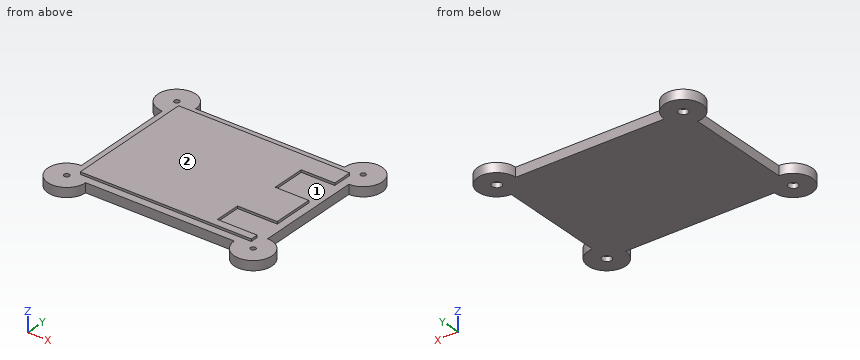
```python
from build123d import *

# Parameters (mm, degrees)
SKETCH024_W     = 79
SKETCH024_H     = 61
PAD006_DEPTH    = 4
SKETCH025_W     = 72.5
SKETCH025_H     = 54.5
PAD007_DEPTH    = 1
SKETCH026_W     = 14.223953
SKETCH026_H     = 14.414499
SKETCH026_W_2   = 16.850891
SKETCH026_H_2   = 11.145231
POCKET015_DEPTH = 1
SKETCH029_R     = 8
PAD010_DEPTH    = 4
SKETCH030_R     = 1.1
POCKET016_DEPTH = 5.001
SKETCH031_R     = 2
POCKET017_DEPTH = 2


with BuildPart() as part:
    # Sketch024 → Pad006 (new body)
    with BuildSketch(Plane.XY):
        Rectangle(SKETCH024_W, SKETCH024_H)
    extrude(amount=-PAD006_DEPTH)

    # Sketch025 (on Face5 of Pad006) → Pad007 (join)
    with BuildSketch(Plane.XY):
        Rectangle(SKETCH025_W, SKETCH025_H)
    extrude(amount=PAD007_DEPTH)

    # Sketch026 (on Face11 of Pad007) → Pocket015 (cut)
    with BuildSketch(Plane.XY.offset(1)):
        with Locations((29.1380235, 11.7657555)):
            Rectangle(SKETCH026_W, SKETCH026_H)
        with Locations((27.8245545, -18.4755795)):
            Rectangle(SKETCH026_W_2, SKETCH026_H_2)
    extrude(amount=-POCKET015_DEPTH, mode=Mode.SUBTRACT)

    # Sketch029 (on Face5 of Pocket015) → Pad010 (join)
    with BuildSketch(Plane(origin=(0, 0, -4), x_dir=(1, 0, 0), z_dir=(0, 0, -1))):
        with Locations((39.5, 30.5)):
            Circle(SKETCH029_R)
        with Locations((39.5, -30.5)):
            Circle(SKETCH029_R)
        with Locations((-39.5, -30.5)):
            Circle(SKETCH029_R)
        with Locations((-39.5, 30.5)):
            Circle(SKETCH029_R)
    extrude(amount=-PAD010_DEPTH)

    # Sketch030 (on Face20 of Pad010) → Pocket016 (cut, through all)
    with BuildSketch(Plane(origin=(0, 0, -4), x_dir=(1, 0, 0), z_dir=(0, 0, -1))):
        with Locations((39.5, 30.5)):
            Circle(SKETCH030_R)
        with Locations((39.5, -30.5)):
            Circle(SKETCH030_R)
        with Locations((-39.5, -30.5)):
            Circle(SKETCH030_R)
        with Locations((-39.5, 30.5)):
            Circle(SKETCH030_R)
    extrude(amount=-POCKET016_DEPTH, mode=Mode.SUBTRACT)

    # Sketch031 (on Face22 of Pocket016) → Pocket017 (cut)
    with BuildSketch(Plane(origin=(0, 0, -4), x_dir=(1, 0, 0), z_dir=(0, 0, -1))):
        with Locations((-39.5, 30.5)):
            Circle(SKETCH031_R)
        with Locations((-39.5, -30.5)):
            Circle(SKETCH031_R)
        with Locations((39.5, 30.5)):
            Circle(SKETCH031_R)
        with Locations((39.5, -30.5)):
            Circle(SKETCH031_R)
    extrude(amount=-POCKET017_DEPTH, mode=Mode.SUBTRACT)


with BuildPart() as part_1:
    # Body002 placement: moved
    add(part.part.moved(Location((0, 0, -17))))


solid = part_1.part
```
Design review of the part built by this model. Coordinates are the model's own, in mm. Face numbers are marked on the shaded views. Coordinates: 2 decimals unless noted, no trailing zeros. Order: outer loops, then holes, each group sorted by start corner. A loop starts at its lowest first (then second) coordinate and runs counter-clockwise, first axis right, second up.
1) Clearance check with flat-ended pins moving along their axes: pin 1 (1.1 mm diameter, centred on y = -0.5, z = -16.5, fed in from +X); pin 2 (0.5 mm diameter, centred on y = -9, z = -16.5, fed in from -X); pin 3 (3 mm diameter, centred on y = 3, z = -19.5, fed in from -X). State where each tip first meets the part, or that it passes through.
2) Wall thickness on line 1 along X through (y, z) = (6.5, -20); line 2 along Y through (x, z) = (14.5, -17.15); line 3 along Z through (x, y) = (-37.5, 23): over which ranges is each line inside the solid? List them lowest first.
3) Mouldability with a two-part tool opening along Y and no side actions: class the marked faces 1 and 2 as +Y half, -Y half, draft (parallel to the pull), parting line (faces both ways), or undercut.
4) Take a section at B-B, the plane x = 20.5. Give the boundary of the cut face in (y, z), and give its area (3 significant figures).
5) Take a section at C-C, the plane y = -19.5. Give the boundary of the cut face in (x, z).
6) Take a section at A-A, the plane y = -11.5. Give the boundary of the cut face in (x, z), and give its area (4 significant figures).
Returned:
1. pin 1: stops at x = 39.5
1. pin 2: stops at x = -36.25
1. pin 3: stops at x = -39.5
2. line 1: x = -39.5 to 39.5
2. line 2: y = -30.5 to 30.5
2. line 3: z = -21 to -17
3. face 1: undercut
3. face 2: draft
4. outline: (-30.5, -21) - (30.5, -21) - (30.5, -17) - (27.25, -17) - (27.25, -16) - (-12.9, -16) - (-12.9, -17) - (-24.05, -17) - (-24.05, -16) - (-27.25, -16) - (-27.25, -17) - (-30.5, -17) - close
4. area: 287 mm2
5. outline: (-39.5, -21) - (39.5, -21) - (39.5, -17) - (19.4, -17) - (19.4, -16) - (-36.25, -16) - (-36.25, -17) - (-39.5, -17) - close
6. outline: (-39.5, -21) - (39.5, -21) - (39.5, -17) - (36.25, -17) - (36.25, -16) - (-36.25, -16) - (-36.25, -17) - (-39.5, -17) - close
6. area: 388.5 mm2
